Source: CAD feature listing. Evaluate the final solid. Frame: model axes, mm. Face numbers are marked on the shaded views. A direction names the side the tool comes from. Give positions to 0.01 mm unless a question says otherwise; leave off trailing zeros. Order: outer loops, then holes, each group sorted by start corner. A loop starts at its lowest first (then second) coordinate and runs counter-clockwise, first axis right, second up. Notation, with made-up numbers: M 64,10 L 99,10 A10 ccw 99,23 Z; hole C 19,38.5 d2. An arc over 180 degrees is marked long. Answer as a JSON object with one key per item and string values. Group by question number.
1. Section query D-D (x = 0). Output: boundary loops of the cut face in (y, z).
2. Section query C-C (y = 9.25). Output: boundary loops of the cut face in (x, z) (3 decimals), plus the area to 3 significant figures.
3. Set-up query: the marked faces 1, 2 and 3. Return all of +Z, -Z, +X, -X, +Y, -Y with unobstructed straight access to the full face (end or side cutting, diameter ignored); none if empty.
4. Pull-direction query (X, two-part tool) for the marked faces 4, 5, 6 and 7; classes: +X half, -X half, draft (parallel to the pull), parting line (faces both ways), or undercut.
5. Pin query (flat end, axial travel): P1, Ø2, axis at x = -27, z = 1.5, coming from the -Y side; P2, Ø3, axis at y = 13.5, z = -5.5, coming from the -X side; P3, Ø10, axis at y = 8.5, z = 12, coming from the -X side; P4, Ø6, axis at x = -33.5, z = 7.5, coming from the +Y side. Return the tip coordinate at first contact, or that it passes through.
6. Section query A-A (z = 0). Output: boundary loops of the cut face in (x, y).
7. Material intervals for L1, parallel to X at y = 7.5, z = 0; L2, parallel to X at y = 2.75, z = 6.75; L3, parallel to X at y = 26.25, z = 0, sorted ascending. Write a range as [from, to].
8. Section query B-B (x = -29). Output: boundary loops of the cut face in (y, z).
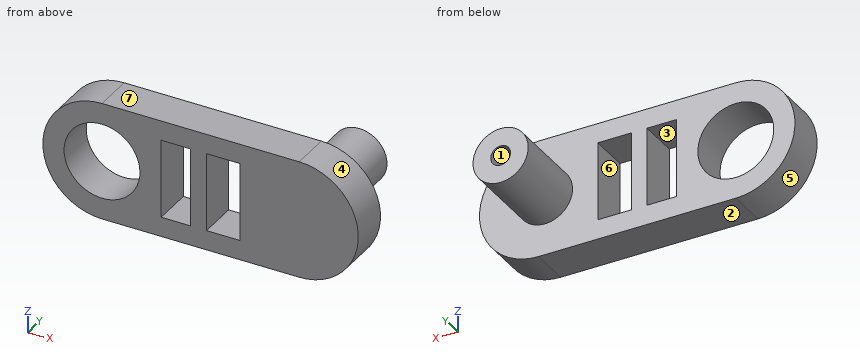
from build123d import *

# Parameters (mm, degrees)
SKETCH1_R           = 9.625
BOSS_EXTRUDE1_DEPTH = 10
SKETCH2_W           = 20
SKETCH2_H           = 20
CUT_EXTRUDE1_DEPTH  = 66.913290189
BOSS_EXTRUDE2_REACH = 70.881
SKETCH4_W           = 4
SKETCH4_H           = 10
SKETCH5_R           = 7
BOSS_EXTRUDE3_DEPTH = 20
SKETCH8_R           = 2.5
CUT_EXTRUDE2_DEPTH  = 10


with BuildPart() as part:
    # Sketch1 → Boss-Extrude1 (new body)
    with BuildSketch(Plane(origin=(0, 0, 0), x_dir=(1, 0, 0), z_dir=(0, 1, 0))):
        with BuildLine():
            Line((-48.400014381, 15), (1.599985619, 15))
            ThreePointArc((1.599985619, 15), (16.599985619, 0), (1.599985619, -15))
            Line((1.599985619, -15), (-48.400014381, -15))
            ThreePointArc((-48.400014381, -15), (-63.400014381, 0), (-48.400014381, 15))
        make_face()
        with Locations(Location((-48.400014381, 0, 0), (0, 0, 270))):
            Circle(SKETCH1_R, mode=Mode.SUBTRACT)
    extrude(amount=BOSS_EXTRUDE1_DEPTH)

    # Sketch2 → Cut-Extrude1 (cut, through all)
    with BuildSketch(Plane(origin=(0, 10, 0), x_dir=(1, 0, 0), z_dir=(0, 1, 0))):
        with Locations((-23.400014381, 0)):
            Rectangle(SKETCH2_W, SKETCH2_H)
    extrude(amount=-CUT_EXTRUDE1_DEPTH, mode=Mode.SUBTRACT)

    # Sketch4 → Boss-Extrude2 (add, up to next)
    with BuildSketch(Plane.XY.offset(-10), mode=Mode.PRIVATE) as boss_extrude2_sk1:
        with Locations((-23.900014381, 5)):
            Rectangle(SKETCH4_W, SKETCH4_H)
    boss_extrude2_tool1 = extrude(boss_extrude2_sk1.sketch, amount=BOSS_EXTRUDE2_REACH, mode=Mode.PRIVATE) - part.part
    add(boss_extrude2_tool1.solids().sort_by_distance((-23.900014, 5, -10))[0])

    # Sketch5 → Boss-Extrude3 (add)
    with BuildSketch(Plane(origin=(0, 10, 0), x_dir=(1, 0, 0), z_dir=(0, 1, 0))):
        with Locations(Location((0, 0, 0), (0, 0, 270))):
            Circle(SKETCH5_R)
    extrude(amount=BOSS_EXTRUDE3_DEPTH)

    # Sketch8 → Cut-Extrude2 (cut)
    with BuildSketch(Plane(origin=(0, 30, 0), x_dir=(1, 0, 0), z_dir=(0, 1, 0))):
        with Locations(Location((0, 0, 0), (0, 0, 270))):
            Circle(SKETCH8_R)
    extrude(amount=-CUT_EXTRUDE2_DEPTH, mode=Mode.SUBTRACT)


solid = part.part
Answer sheet:
{
 "1": {"outline": "M 0,-15 L 10,-15 L 10,-7 L 30,-7 L 30,-2.5 L 20,-2.5 L 20,2.5 L 30,2.5 L 30,7 L 10,7 L 10,15 L 0,15 Z"},
 "2": {"outline": "M -48.4,-15 L 1.6,-15 A15 ccw 1.6,15 L -48.4,15 A15 ccw Z; hole C -48.4,0 d19.25; hole M -33.4,-10 L -25.9,-10 L -25.9,10 L -33.4,10 Z; hole M -21.9,-10 L -13.4,-10 L -13.4,10 L -21.9,10 Z", "area": "1,600 mm^2"},
 "3": {"face 1": "+Y", "face 2": "-Z, +X, -X, +Y, -Y", "face 3": "+Y, -Y"},
 "4": {"face 4": "+X half", "face 5": "-X half", "face 6": "undercut", "face 7": "draft"},
 "5": {"P1": "through", "P2": "x = -5.74", "P3": "x = -61.67", "P4": "y = 10"},
 "6": {"outline": "M -63.4,0 L -58.03,0 L -58.03,10 L -63.4,10 Z; M -38.78,0 L -33.4,0 L -33.4,10 L -38.78,10 Z; M -25.9,0 L -21.9,0 L -21.9,10 L -25.9,10 Z; M -13.4,0 L 16.6,0 L 16.6,10 L 7,10 L 7,30 L 2.5,30 L 2.5,20 L -2.5,20 L -2.5,30 L -7,30 L -7,10 L -13.4,10 Z"},
 "7": {"L1": "[-63.4, -58.03], [-38.78, -33.4], [-25.9, -21.9], [-13.4, 16.6]", "L2": "[-61.8, -55.26], [-41.54, -33.4], [-25.9, -21.9], [-13.4, 15]", "L3": "[-7, -2.5], [2.5, 7]"},
 "8": {"outline": "M 0,-15 L 10,-15 L 10,-10 L 0,-10 Z; M 0,10 L 10,10 L 10,15 L 0,15 Z"}
}
